CAD build for the part. Positions are in the model's coordinates, mm. A direction names the side the tool comes from. Coordinates: 2 decimals unless noted, no trailing zeros. Loops run counter-clockwise (first coordinate to the right, second up) from the corner with the lowest first, then second, coordinate; pieces in that order, holes last.
1) Wall check: line 1 along X through (y, z) = (1.75, 56.1); line 2 along Z through (x, y) = (0, 1.1); line 3 along Z through (x, y) = (6.5, -2.7). Give the ranges that are in metal, low to high.
2) Saw through at D-D, the plane z = 8.5. Write the cut outline in (x, y).
3) Saw through at C-C, the plane x = 5.5. Write the cut outline in (y, z), and give its area (3 significant figures).
4) Which spindle directions (+Z, -Z, +X, -X, +Y, -Y) get a long thin tool onto all of the face, cutting with end or side? Do faces 1 (the flat face through (6.2, 0.5, 29.3)), 2 (the cylindrical face through (10.841, 0.24, 51.497)), 3 (the flat face through (10.2, 1.5, 17.5)). Say none if no direction does.
5) Saw through at A-A, the plane z = 27.5. Write the cut outline in (x, y), and give its area (3 significant figures).
6) Pin check, flat tips, straight feed: pin 1 Ø1.5 at (x, z) = (-0.5, 17) entering from -Y; pin 2 Ø2 at (y, z) = (0.5, 9.5) entering from -X; pin 3 Ø1.6 at (y, z) = (0, 41.5) entering from +X. Stop position of each tip, or through.
```python
from build123d import *

# Parameters (mm, degrees)
SKETCH_1_R               = 1.35
EXTRUDE_1_DEPTH          = 2
EXTRUDE_2_DEPTH          = 2
CUT_EXTRUDE_1_DEPTH      = 62.421331799
CUT_EXTRUDE_1_DEPTH_BACK = 62.421331799
EXTRUDE_START            = 3.5
EXTRUDE_3_DEPTH          = 3.5
SKETCH_5_W               = 14
SKETCH_5_H               = 4.5
CUT_EXTRUDE_2_DEPTH      = 9
CUT_EXTRUDE_3_REACH      = 63.635
SKETCH_7_W               = 7
SKETCH_7_H               = 24
CUT_EXTRUDE_4_DEPTH      = 62.488454201
CHAMFER_1_SIZE           = 1
EXTRUDE_4_DEPTH          = 3
EXTRUDE_START_2          = 3
EXTRUDE_5_DEPTH          = 3
CHAMFER_2_SIZE           = 1.5
EXTRUDE_6_DEPTH          = 1
EXTRUDE_START_3          = 1
EXTRUDE_7_DEPTH          = 1
SKETCH_12_R              = 3
CUT_EXTRUDE_5_DEPTH      = 0.5


with BuildPart() as part:
    # 草图1 → 凸台-拉伸1 (new body)
    with BuildSketch(Plane(origin=(0, 0, 0), x_dir=(1, 0, 0), z_dir=(0, 1, 0))):
        with BuildLine():
            Line((0, 3.3), (11.7, 3.3))
            ThreePointArc((11.7, 3.3), (13.538477631, 2.538477631), (14.3, 0.7))
            Line((14.3, 0.7), (14.3, -59.7))
            Line((14.3, -59.7), (-3.3, -59.7))
            Line((-3.3, -59.7), (-3.3, 0))
            Line((-3.3, 0), (-3.3, 3.3))
            Line((-3.3, 3.3), (0, 3.3))
        make_face()
        with Locations(Location((0, 0, 0), (0, 0, 270))):
            Circle(SKETCH_1_R, mode=Mode.SUBTRACT)
        with Locations(Location((10.7, -56.1, 0), (0, 0, 270))):
            Circle(SKETCH_1_R, mode=Mode.SUBTRACT)
    extrude(amount=EXTRUDE_1_DEPTH)

    # 草图2 → 凸台-拉伸2 (add)
    with BuildSketch(Plane(origin=(0, 2, 0), x_dir=(1, 0, 0), z_dir=(0, 1, 0))):
        Polygon((-3.3, 1.179910787), (-6.171573065, -59.7), (-3.3, -59.7), align=None)
    extrude(amount=-EXTRUDE_2_DEPTH)

    # 草图3 → 切除-拉伸1 (cut, two sides: drawn at the far end of the back side and taken through both)
    with BuildSketch(Plane(origin=(0, 2, 0), x_dir=(1, 0, 0), z_dir=(0, 1, 0)).offset(-CUT_EXTRUDE_1_DEPTH_BACK)):
        Polygon((-3.3, 3.3), (-3.3, 1.179910787), (-3.2, 3.3), align=None)
        with BuildLine():
            ThreePointArc((-2.499988961, -59.7), (-4.984483511, -58.608076588), (-6.001389, -56.091946))
            Line((-6.001389, -56.091946), (-6.171573065, -59.7))
            Line((-6.171573065, -59.7), (-2.499988961, -59.7))
        make_face()
    extrude(amount=CUT_EXTRUDE_1_DEPTH + CUT_EXTRUDE_1_DEPTH_BACK, mode=Mode.SUBTRACT)

    # 草图4 → 凸台-拉伸3 (add)
    with BuildSketch(Plane.XZ.offset(EXTRUDE_START)):
        with BuildLine():
            Line((-6.001389, 56.091946), (-3.2, -3.3))
            Line((-3.2, -3.3), (11.7, -3.3))
            ThreePointArc((11.7, -3.3), (13.538477631, -2.538477631), (14.3, -0.7))
            Line((14.3, -0.7), (14.3, 59.7))
            Line((14.3, 59.7), (-2.499988961, 59.7))
            ThreePointArc((-2.499988961, 59.7), (-4.984483511, 58.608076588), (-6.001389, 56.091946))
        make_face()
        with BuildLine():
            Line((12.8, -0.7), (12.8, 54.32447191))
            ThreePointArc((12.8, 54.32447191), (12.644543648, 58.044543648), (8.92447191, 58.2))
            Line((8.92447191, 58.2), (-2.476371899, 58.2))
            ThreePointArc((-2.476371899, 58.2), (-3.904150356, 57.567435732), (-4.501255338, 56.124468472))
            Line((-4.501255338, 56.124468472), (-1.945653662, 1.943433001))
            ThreePointArc((-1.945653662, 1.943433001), (-1.872904729, -2.013635488), (2.079062289, -1.8))
            Line((2.079062289, -1.8), (11.7, -1.8))
            ThreePointArc((11.7, -1.8), (12.477817459, -1.477817459), (12.8, -0.7))
        make_face(mode=Mode.SUBTRACT)
    extrude(amount=-EXTRUDE_3_DEPTH)

    # 草图5 → 切除-拉伸2 (cut)
    with BuildSketch(Plane(origin=(14.3, 0, 0), x_dir=(0, 0, -1), z_dir=(1, 0, 0))):
        with Locations((-42.2, -1.25)):
            Rectangle(SKETCH_5_W, SKETCH_5_H)
    extrude(amount=-CUT_EXTRUDE_2_DEPTH, mode=Mode.SUBTRACT)

    # 切除-拉伸3: up to this face of the body (flat: up to its plane)
    cut_extrude_3_end = Plane(part.part.faces().sort_by_distance((9.8, 1, 42.2))[0])
    # 草图6 → 切除-拉伸3 (cut, up to the picked face)
    with BuildSketch(Plane.XZ.offset(3.5), mode=Mode.PRIVATE) as cut_extrude_3_sk1:
        with BuildLine():
            Line((2.158571571, 33.539745962), (2.158571571, 50.860254038))
            ThreePointArc((2.158571571, 50.860254038), (17.158571571, 42.2), (2.158571571, 33.539745962))
        make_face()
    cut_extrude_3_tool1 = split(extrude(cut_extrude_3_sk1.sketch, amount=-CUT_EXTRUDE_3_REACH, mode=Mode.PRIVATE), bisect_by=cut_extrude_3_end, keep=Keep.BOTH, mode=Mode.PRIVATE)
    add(cut_extrude_3_tool1.solids().sort_by(Axis((8.87184, -3.5, 42.2), (0, 1, 0)))[0], mode=Mode.SUBTRACT)

    # 草图7 → 切除-拉伸4 (cut, through all)
    with BuildSketch(Plane.XZ):
        with Locations((6.2, 17.3)):
            Rectangle(SKETCH_7_W, SKETCH_7_H)
    extrude(amount=-CUT_EXTRUDE_4_DEPTH, mode=Mode.SUBTRACT)

    # 倒角1
    chamfer_1_edges = [part.edges().sort_by_distance(p)[0] for p in [
        (2.7, 2, 17.3),
        (6.2, 2, 29.3),
        (9.7, 2, 17.3),
        (6.2, 2, 5.3),
    ]]
    chamfer(chamfer_1_edges, length=CHAMFER_1_SIZE)

    # 草图8 → 凸台-拉伸4 (add)
    with BuildSketch(Plane.XZ):
        Polygon((-2.891678333, 22), (0.3, 22), (0.3, 18), (-2.703007027, 18), align=None)
        Polygon((-2.514335721, 14), (0.3, 14), (0.3, 10), (-2.325664416, 10), align=None)
    extrude(amount=EXTRUDE_4_DEPTH)

    # 草图9 → 凸台-拉伸5 (add)
    with BuildSketch(Plane.XZ.offset(EXTRUDE_START_2)):
        with BuildLine():
            Line((2.75, 0), (2.75, 2.6))
            Line((2.75, 2.6), (3.3, 2.6))
            Line((3.3, 2.6), (3.3, -1.8))
            Line((3.3, -1.8), (2.079062289, -1.8))
            ThreePointArc((2.079062289, -1.8), (2.576812109, -0.960489122), (2.75, 0))
        make_face()
    extrude(amount=-EXTRUDE_5_DEPTH)

    # 倒角2
    chamfer_2_edges = [part.edges().sort_by_distance(p)[0] for p in [
        (0.3, -3, 20),
        (0.3, -3, 12),
        (3.025, -3, 2.6),
    ]]
    chamfer(chamfer_2_edges, length=CHAMFER_2_SIZE)

    # 草图10 → 凸台-拉伸6 (add)
    with BuildSketch(Plane.XZ):
        Polygon((0.3, 22), (0.3, 31.6), (-3.344489466, 31.6), (-2.891678333, 22), align=None)
        Polygon((0.3, 18), (0.3, 14), (-2.514335721, 14), (-2.703007027, 18), align=None)
    extrude(amount=EXTRUDE_6_DEPTH)

    # 草图11 → 凸台-拉伸7 (add)
    with BuildSketch(Plane.XZ.offset(EXTRUDE_START_3)):
        with BuildLine():
            Line((0.3, 31.6), (12.8, 31.6))
            Line((12.8, 31.6), (12.8, 33.943227914))
            ThreePointArc((12.8, 33.943227914), (7.537460775, 32.207180429), (2.158571571, 33.539745962))
            Line((2.158571571, 33.539745962), (2.158571571, 33.6))
            Line((2.158571571, 33.6), (-3.438825119, 33.6))
            Line((-3.438825119, 33.6), (-3.344489466, 31.6))
            Line((-3.344489466, 31.6), (0.3, 31.6))
        make_face()
    extrude(amount=-EXTRUDE_7_DEPTH)

    # 草图12 → 切除-拉伸5 (cut)
    with BuildSketch(Plane(origin=(0, 2, 0), x_dir=(1, 0, 0), z_dir=(0, 1, 0))):
        with Locations(Location((0, 0, 0), (0, 0, 270))):
            Circle(SKETCH_12_R)
        with Locations(Location((10.7, -56.1, 0), (0, 0, 270))):
            Circle(SKETCH_12_R)
    extrude(amount=-CUT_EXTRUDE_5_DEPTH, mode=Mode.SUBTRACT)

    # 倒角3
    # the kernel refuses this chamfer: 0.75 mm, written as the material it takes off along each edge
    with BuildSketch(Plane(origin=(10.7, -3.5, 56.1), x_dir=(-0.7048818539423597, 0, -0.7093247295722755), z_dir=(-0.7093247295722755, 0, 0.7048818539423597))) as chamfer_3_piece_1:
        with BuildLine():
            Line((3.521213203, 0.021213203), (2.728786797, -0.771213203))
            Line((2.728786797, -0.771213203), (2.713786797, -0.771213203))
            ThreePointArc((2.713786797, -0.771213203), (2.735, -0.385606602), (2.735, 0))
            Line((2.735, 0), (2.75, 0.015))
            ThreePointArc((2.75, 0.015), (3.135606602, 0.015), (3.521213203, 0.036213203))
            Line((3.521213203, 0.036213203), (3.521213203, 0.021213203))
        make_face()
    revolve(axis=Axis((10.7, -3.5, 56.1), (0, -1, 0)), revolution_arc=359.64, mode=Mode.SUBTRACT)
    with BuildSketch(Plane(origin=(0, -3.5, 0), x_dir=(0.6787525361233852, 0, 0.7343670708209028), z_dir=(0.7343670708209028, 0, -0.6787525361233852))) as chamfer_3_piece_2:
        with BuildLine():
            Line((2.728786797, -0.771213203), (3.521213203, 0.021213203))
            Line((3.521213203, 0.021213203), (3.521213203, 0.036213203))
            ThreePointArc((3.521213203, 0.036213203), (3.135606602, 0.015), (2.75, 0.015))
            Line((2.75, 0.015), (2.735, 0))
            ThreePointArc((2.735, 0), (2.735, -0.385606602), (2.713786797, -0.771213203))
            Line((2.713786797, -0.771213203), (2.728786797, -0.771213203))
        make_face()
    revolve(axis=Axis((0, -3.5, 0), (0, -1, 0)), revolution_arc=359.64, mode=Mode.SUBTRACT)


solid = part.part
```
Data:
1. line 1: x = -6 to 7.7, 13.7 to 14.3
1. line 2: z = -3.3 to -1.35, 1.35 to 59.7
1. line 3: z = -3.3 to -1.8, 58.2 to 59.7
2. outline: (-3.76, -3.5) - (-2.25, -3.5) - (-2.25, 0) - (2.7, 0) - (2.7, 1) - (1.7, 2) - (-3.76, 2) - close; (9.7, 0) - (12.8, 0) - (12.8, -3.5) - (14.3, -3.5) - (14.3, 2) - (10.7, 2) - (9.7, 1) - close
3. outline: (-3.5, -3.3) - (2, -3.3) - (2, 4.3) - (1, 5.3) - (0, 5.3) - (0, -1.8) - (-3.5, -1.8) - close; (-3.5, 58.2) - (0, 58.2) - (0, 52.06) - (1, 52.06) - (1, 32.34) - (-1, 32.34) - (-1, 31.6) - (0, 31.6) - (0, 29.3) - (1, 29.3) - (2, 30.3) - (2, 59.7) - (-3.5, 59.7) - close
3. area: 68.5 mm2
4. face 1: +Y, -Y
4. face 2: -Y
4. face 3: +Y
5. outline: (-4.65, -3.5) - (-3.15, -3.5) - (-3.15, -1) - (0.3, -1) - (0.3, 0) - (2.7, 0) - (2.7, 1) - (1.7, 2) - (-4.65, 2) - close; (9.7, 0) - (12.8, 0) - (12.8, -3.5) - (14.3, -3.5) - (14.3, 2) - (10.7, 2) - (9.7, 1) - close
5. area: 36.9 mm2
6. pin 1: stops at y = -1
6. pin 2: stops at x = -3.85
6. pin 3: stops at x = 2.16
